The model under review builds one solid part; all positions refer to its coordinate system, in mm. Face numbers are marked on the shaded views. A direction names the side the tool comes from. Round coordinates to 2 decimals unless told otherwise and drop trailing zeros. Loops run counter-clockwise (first coordinate to the right, second up) from the corner with the lowest first, then second, coordinate; pieces in that order, holes last. Notation, with made-up numbers: (86, 66) -> (108, 66) arc R23 cw to (108, 79) -> close; hole circle Ø2 at (12.25, 33.5). An arc over 180 degrees is marked (long way). Use CSV: the item, a comma, the result in double quotes. Start each with the question number.
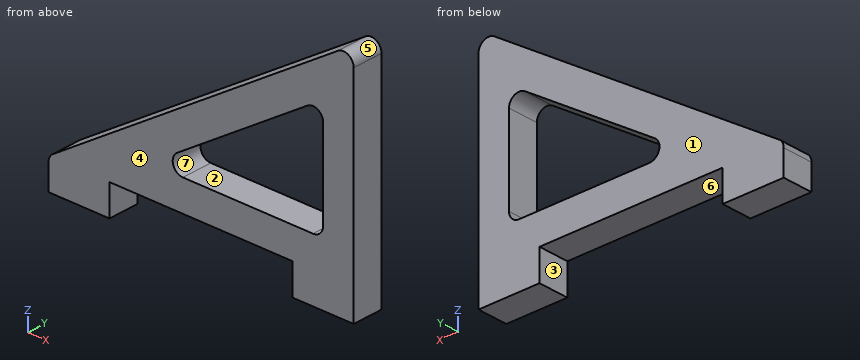
```python
from build123d import *

# Parameters (mm, degrees)
SKETCH1_W           = 6
SKETCH1_H           = 3
BOSS_EXTRUDE1_DEPTH = 3
CUT_EXTRUDE1_REACH  = 28.387
FILLET1_R           = 1


with BuildPart() as part:
    # Sketch1 → Boss-Extrude1 (new body)
    with BuildSketch(Plane(origin=(0, 0, 0), x_dir=(1, 0, 0), z_dir=(0, 1, 0))):
        Polygon((-15, -1.5), (15, -21.5), (15, -1.5), align=None)
        with Locations((-12, 0)):
            Rectangle(SKETCH1_W, SKETCH1_H)
        with Locations((12, 0)):
            Rectangle(SKETCH1_W, SKETCH1_H)
    extrude(amount=BOSS_EXTRUDE1_DEPTH)

    # Sketch2 → Cut-Extrude1 (cut, up to next)
    with BuildSketch(Plane(origin=(0, 3, 0), x_dir=(1, 0, 0), z_dir=(0, 1, 0)), mode=Mode.PRIVATE) as cut_extrude1_sk1:
        Polygon((12, -15.894448725), (-5.091673087, -4.5), (12, -4.5), align=None)
    cut_extrude1_tool1 = extrude(cut_extrude1_sk1.sketch, amount=-CUT_EXTRUDE1_REACH, mode=Mode.PRIVATE) & part.part
    add(cut_extrude1_tool1.solids().sort_by_distance((6.302776, 3, 8.29815))[0], mode=Mode.SUBTRACT)

    # Fillet1
    fillet1_edges = [part.edges().sort_by_distance(p)[0] for p in [
        (-15, 1.5, 1.5),
        (15, 1.5, 21.5),
        (12, 1.5, 15.894448725),
        (-5.091673087, 1.5, 4.5),
        (12, 1.5, 4.5),
    ]]
    fillet(fillet1_edges, radius=FILLET1_R)


solid = part.part
```
1. The part is to be moulded in two halves that separate along Z. For the marked faces 4, 5, 6 and 7, say which applies: pulls with the +Z half, pulls with the -Z half, needs draft (parallel to the pull), parting line crosses it, or undercut.
2. For the marked faces 1, 2 and 3, list the 3-axis set-ups (+Z, -Z, +X, -X, +Y, -Y) from which the entire face can be reached by the end or side of a thin tool; tool diameter is ignored.
3. Take a section at A-A, the plane y = 1. Give the boundary of the cut face in (x, z).
4. Clearance check with flat-ended pins moving along their axes: P1, Ø0.9, axis at y = 1.5, z = 10.5, coming from the -X side (3 decimals); P2, Ø1.5, axis at x = -3.5, y = 1, coming from the -Z side; P3, Ø0.9, axis at x = 5.5, y = 1, coming from the +Z side; P4, Ø4, axis at x = -11.5, z = 7.5, coming from the +Y side. State where each tip first meets the part, or that it passes through.
5. For line 1 along X through (y, z) = (1.3, 5.5); line 2 along X through (y, z) = (2.8, -0.25); line 3 along Z through (x, y) = (-2.5, 2.7), list the stretches that pass through material, from the lowest coordinate up. Write a range as from..to.
6. Take a section at C-C, the plane x = 3. Give the boundary of the cut face in (y, z).
7. Take a section at D-D, the plane x = -8. Give the boundary of the cut face in (y, z), then the cut area to 3 significant figures.
8. Take a section at B-B, the plane z = 0.5. Give the boundary of the cut face in (x, y), then the cut area to 3 significant figures.
Results:
1,face 4,"needs draft"
1,face 5,"pulls with the +Z half"
1,face 6,"pulls with the -Z half"
1,face 7,"undercut"
2,face 1,"+Z, -Z, +X, -X, +Y"
2,face 2,"+Y, -Y"
2,face 3,"-Z, +Y, -Y"
3,outline,"(-15, -1.5) -> (-9, -1.5) -> (-9, 1.5) -> (9, 1.5) -> (9, -1.5) -> (15, -1.5) -> (15, 19.63) arc R1 ccw to (13.45, 20.46) -> (-14.55, 1.8) arc R1 ccw to (-15, 0.96) -> close; hole (-2.34, 6.33) arc R1 ccw to (-1.79, 4.5) -> (11, 4.5) arc R1 ccw to (12, 5.5) -> (12, 14.03) arc R1 ccw to (10.45, 14.86) -> close"
4,P1,"x = -2.175"
4,P2,"z = 1.5"
4,P3,"z = 15.47"
4,P4,"through"
5,line 1,"-9..-2.79, 12..15"
5,line 2,"-15..-9, 9..15"
5,line 3,"1.5..4.8, 6.2..9.83"
6,outline,"(0, 1.5) -> (3, 1.5) -> (3, 4.5) -> (0, 4.5) -> close; (0, 9.89) -> (3, 9.89) -> (3, 13.5) -> (0, 13.5) -> close"
7,outline,"(0, 1.5) -> (3, 1.5) -> (3, 6.17) -> (0, 6.17) -> close"
7,area,"14.0 mm²"
8,outline,"(-15, 0) -> (-9, 0) -> (-9, 3) -> (-15, 3) -> close; (9, 0) -> (15, 0) -> (15, 3) -> (9, 3) -> close"
8,area,"36.0 mm²"
